Can you work these out from the model? Positions are in its coordinate system, mm. A direction names the side the tool comes from. Round coordinates to 2 decimals unless told otherwise and drop trailing zeros. Write each loop counter-clockwise with the first axis right and the second up, starting at its lowest first coordinate (ties: lowest second). Pieces come first, ordered by that corner, then holes.
Q1. Please list where these lines run through material, in increasing order: line 1 along Z through (x, y) = (34, 91.5); line 2 along X through (y, z) = (83.5, 18); line 3 along Y through (x, z) = (-69, 63).
Q2. If we section it at A-A (x = 17): Please give me the cut outline in (y, z), plus the area to 3 significant figures.
Q3. We'd pull the mould along Z, two halves only. Please class faces 1 (the cylindrical face through (20.265, 86.622, -134.173)), 2 (the flat face through (79, 56, 62.981)), 3 (the cylindrical face through (146.446, 13.804, 84.657)), 4 (the flat face through (43, 84, 23)): +Z half, -Z half, draft (parallel to the pull), parting line (faces both ways), or undercut.
Q4. For faces 5 (the flat face through (34.336, 44, 77)), 6 (the flat face through (104.336, 62, 9)), 7 (the flat face through (44, 54, -31)), which set-ups out of +Z, -Z, +X, -X, +Y, -Y let a thin tool reach every point of the face, with its end or its side?
Q5. If we section it at C-C (y = 22): Please give me the cut outline in (x, z), plus the area to 3 significant figures.
Q6. I'm going to push flat-ended pins straight in: pin 1 Ø4 at (x, y) = (10.5, 58.5) entering from +Z; pin 2 Ø24 at (x, z) = (130, 64) entering from +Y; pin 3 Ø6 at (x, z) = (106, 14) entering from -Y. Where does each tip first touch, or does it pass through?
Q7. If we section it at B-B (z = -94.5): Please give me the cut outline in (x, y).
Q8. If we section it at D-D (z = 66.5): Please give me the cut outline in (x, y), plus the area to 3 significant figures.
from build123d import *

# Parameters (mm, degrees)
SKETCH_1_R          = 18
EXTRUDE_1_DEPTH     = 28
SKETCH_2_W          = 121.577423065
SKETCH_2_H          = 141
EXTRUDE_2_DEPTH     = 56
SKETCH_5_W          = 113
SKETCH_5_H          = 26
CUT_EXTRUDE_1_DEPTH = 180
SKETCH_7_R          = 60.788711533
SKETCH_7_R_2        = 35
EXTRUDE_4_DEPTH     = 54
EXTRUDE_START       = -70
EXTRUDE_5_DEPTH     = 20
CUT_EXTRUDE_START   = -20
SKETCH_9_R          = 35
CUT_EXTRUDE_2_DEPTH = 20
CUT_EXTRUDE_5_DEPTH = 236.915979109


with BuildPart() as part:
    # 스케치1 → 보스-돌출1 (new body)
    with BuildSketch(Plane(origin=(0, 0, 0), x_dir=(1, 0, 0), z_dir=(0, 1, 0))):
        with BuildLine():
            Line((-48.732108463, -34.980719949), (131.267891537, -34.980719949))
            ThreePointArc((131.267891537, -34.980719949), (171.267891537, -74.980719949), (131.267891537, -114.980719949))
            Line((131.267891537, -114.980719949), (-48.732108463, -114.980719949))
            ThreePointArc((-48.732108463, -114.980719949), (-88.732108463, -74.980719949), (-48.732108463, -34.980719949))
        make_face()
        with Locations(Location((-48.732108463, -74.980719949, 0), (0, 0, 270))):
            Circle(SKETCH_1_R, mode=Mode.SUBTRACT)
        with Locations(Location((131.267891537, -74.980719949, 0), (0, 0, 270))):
            Circle(SKETCH_1_R, mode=Mode.SUBTRACT)
    extrude(amount=EXTRUDE_1_DEPTH)

    # 스케치2 → 보스-돌출2 (add)
    with BuildSketch(Plane(origin=(0, 28, 0), x_dir=(1, 0, 0), z_dir=(0, 1, 0))):
        with Locations((43.54746822, 7.519280051)):
            Rectangle(SKETCH_2_W, SKETCH_2_H)
    extrude(amount=EXTRUDE_2_DEPTH)

    # 스케치5 → 컷-돌출1 (cut)
    with BuildSketch(Plane(origin=(104.336179752, 0, 0), x_dir=(0, 0, -1), z_dir=(1, 0, 0))):
        with Locations((21.519280051, 41)):
            Rectangle(SKETCH_5_W, SKETCH_5_H)
    extrude(amount=-CUT_EXTRUDE_1_DEPTH, mode=Mode.SUBTRACT)

    # 스케치7 → 보스-돌출4 (add)
    with BuildSketch(Plane.XZ.offset(-54)):
        with Locations(Location((43.54746822, -78.019280051, 0), (0, 0, 270))):
            Circle(SKETCH_7_R)
        with Locations(Location((43.54746822, -78.019280051, 0), (0, 0, 270))):
            Circle(SKETCH_7_R_2, mode=Mode.SUBTRACT)
    extrude(amount=-EXTRUDE_4_DEPTH)

    # 스케치8 → 보스-돌출5 (add)
    with BuildSketch(Plane(origin=(104.336179752, 0, 0), x_dir=(0, 0, -1), z_dir=(1, 0, 0)).offset(EXTRUDE_START)):
        Polygon((-114.980719949, 28), (-62.980719949, 84), (-62.980719949, 28), align=None)
    extrude(amount=EXTRUDE_5_DEPTH)

    # 스케치9 → 컷-돌출2 (cut)
    with BuildSketch(Plane(origin=(0, 84, 0), x_dir=(1, 0, 0), z_dir=(0, 1, 0)).offset(CUT_EXTRUDE_START)):
        with Locations(Location((43.54746822, 78.019280051, 0), (0, 0, 90))):
            Circle(SKETCH_9_R)
    extrude(amount=CUT_EXTRUDE_2_DEPTH, mode=Mode.SUBTRACT)

    # 스케치11 → 컷-돌출5 (cut, through all)
    with BuildSketch(Plane(origin=(0, 84, 0), x_dir=(1, 0, 0), z_dir=(0, 1, 0))):
        with BuildLine():
            Line((78.54746822, 78.019280051), (8.54746822, 78.019280051))
            ThreePointArc((8.54746822, 78.019280051), (43.54746822, 43.019280051), (78.54746822, 78.019280051))
        make_face()
    extrude(amount=-CUT_EXTRUDE_5_DEPTH, mode=Mode.SUBTRACT)


solid = part.part
A:
1. line 1: z = -138.05 to -111.69, -44.35 to -17.99
1. line 2: x = -17.24 to 104.34
1. line 3: y = 0 to 28
2. outline: (0, 34.98) - (54, 34.98) - (54, -55.21) - (108, -55.21) - (108, -23.33) - (84, -23.33) - (84, 62.98) - (28, 62.98) - (28, 114.98) - (0, 114.98) - close; (54, -132.7) - (108, -132.7) - (108, -100.83) - (54, -100.83) - close
2. area: 9,000 mm2
3. face 1: parting line
3. face 2: +Z half
3. face 3: undercut
3. face 4: draft
4. face 5: +Z, -X, +Y
4. face 6: +Z, -Z, +X, +Y
4. face 7: -Z, +X, -X, -Y
5. outline: (-48.73, 34.98) - (131.27, 34.98) arc R40 ccw to (131.27, 114.98) - (-48.73, 114.98) arc R40 ccw to start; hole circle Ø36 at (-48.73, 74.98); hole circle Ø36 at (131.27, 74.98)
5. area: 17,400 mm2
6. pin 1: stops at z = 62.98
6. pin 2: stops at y = 28
6. pin 3: stops at y = 54
7. outline: (-14.96, 54) - (12.67, 54) - (12.67, 108) - (-14.96, 108) - close; (74.42, 54) - (102.06, 54) - (102.06, 108) - (74.42, 108) - close
8. outline: (-87.82, 0) - (-64.61, 0) - (-64.61, 28) - (-87.82, 28) - close; (-32.86, 0) - (115.39, 0) - (115.39, 28) - (54.34, 28) - (54.34, 80.21) - (34.34, 80.21) - (34.34, 28) - (-32.86, 28) - close; (147.14, 0) - (170.36, 0) - (170.36, 28) - (147.14, 28) - close
8. area: 6,500 mm2
